```python
from build123d import *

# Parameters (mm, degrees)
F0_W     = 5.2
F0_H     = 1.8
F0_H_2   = 5.2
F0_R     = 1.35
F1_DEPTH = 3
F2_W     = 5.2
F2_H     = 1.8
F3_DEPTH = 1.8
F4_W     = 7
F4_H     = 7
F4_R     = 1.35
F5_DEPTH = 3
F6_R     = 2.5


with BuildPart() as f1:
    # F0 (on Top) → F1 (new body)
    with BuildSketch(Plane.XY):
        with Locations((-0.1, 3.6)):
            Rectangle(F0_W, F0_H)
        Polygon((-4.5, -2.5), (-2.7, -2.5), (-2.7, 2.7), (-2.7, 4.5), (-4.5, 4.5), align=None)
        with Locations((-0.1, 0.1)):
            Rectangle(F0_W, F0_H_2)
        Circle(F0_R, mode=Mode.SUBTRACT)
    extrude(amount=-F1_DEPTH)

    # F0 (on Top) + F2 (on face) → F3 (join)
    with BuildSketch(Plane.XY):
        Polygon((-4.5, -2.5), (-2.7, -2.5), (-2.7, 2.7), (-2.7, 4.5), (-4.5, 4.5), align=None)
    with BuildSketch(Plane.XY):
        with Locations((-0.1, 3.6)):
            Rectangle(F2_W, F2_H)
    extrude(amount=F3_DEPTH)

    # F4 (on face) → F5 (join)
    with BuildSketch(Plane.XY.offset(1.8)):
        with Locations((-1, 1)):
            Rectangle(F4_W, F4_H)
        Circle(F4_R, mode=Mode.SUBTRACT)
    extrude(amount=F5_DEPTH)

    # F6
    f6_edges = [f1.edges().sort_by_distance(p)[0] for p in [
        (2.5, -2.5, 3.3),
        (2.5, -2.5, -1.5),
    ]]
    fillet(f6_edges, radius=F6_R)


solid = f1.part
```
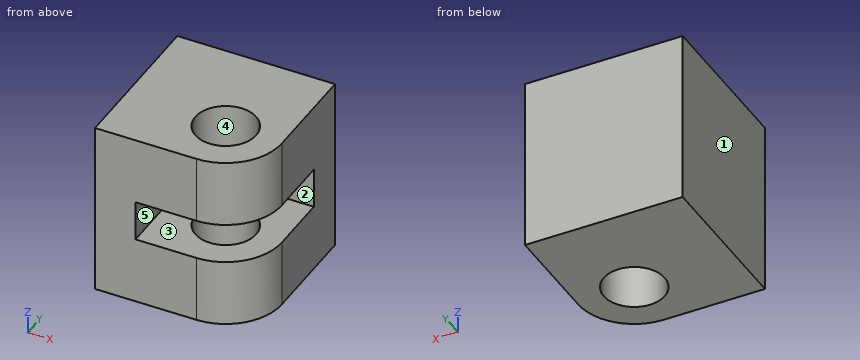
Model file for the job. Use its own axes, mm. Face numbers are marked on the shaded views. A direction names the side the tool comes from. Round coordinates to 2 decimals unless told otherwise and drop trailing zeros. Write each loop counter-clockwise with the first axis right and the second up, starting at its lowest first coordinate (ties: lowest second). Pieces come first, ordered by that corner, then holes. Notation, with made-up numbers: (-6.5, 42) - (34.5, 42) arc R24 ccw to (34.5, 73) - close; hole circle Ø8 at (54, 53.25). An arc over 180 degrees is marked (long way). Use CSV: the item, a comma, the result in double quotes. Start each with the question number.
Item 1: Drill centre lines: L1, parallel to Z at x = 2.25, y = -1; L2, parallel to Y at x = 1.25, z = 1.75; L3, parallel to Y at x = 1, z = 3. Where is each one in solid material? Low to high. Write a range as [from, to].
Item 2: Band-saw the part on C-C (y = 0.75). Write the cut outline in (x, z), and give its area (3 significant figures).
Item 3: Tool access for the marked faces 1 and 2: list every direction of +Z, -Z, +X, -X, +Y, -Y with a clear straight run to the whole face (end or side of a thin tool).
Item 4: Two-plate mould, pull along X, no slides. Class the marked faces 3, 4 and 5: released by +X, released by -X, zero draft, split by the parting line, or undercut.
Item 5: Band-saw the part on D-D (x = 1.5). Write the cut outline in (y, z), and give its area (3 significant figures).
Item 6: Band-saw the part on B-B (x = -0.75). Write the cut outline in (y, z).
Item 7: Band-saw the part on A-A (z = -0.25). Write the cut outline in (x, y), and give its area (3 significant figures).
Item 8: Pin check, flat tips, straight feed: P1, Ø0.9, axis at x = 0, z = 1, coming from the -Y side; P2, Ø0.5, axis at y = 1, z = 1, coming from the +X side. Stop position of each tip, or through.
Checked values:
1,L1,"z = [-3, 0], [1.8, 4.8]"
1,L2,"y = [2.7, 4.5]"
1,L3,"y = [-2.29, -0.91], [0.91, 4.5]"
2,outline,"(-4.5, -3) - (-1.12, -3) - (-1.12, 0) - (-2.7, 0) - (-2.7, 1.8) - (-1.12, 1.8) - (-1.12, 4.8) - (-4.5, 4.8) - close; (1.12, -3) - (2.5, -3) - (2.5, 0) - (1.12, 0) - close; (1.12, 1.8) - (2.5, 1.8) - (2.5, 4.8) - (1.12, 4.8) - close"
2,area,"31.8 mm²"
3,face 1,"+Z, -Z, -X, +Y, -Y"
3,face 2,"+X, -Y"
4,face 3,"zero draft"
4,face 4,"undercut"
4,face 5,"released by +X"
5,outline,"(-2, -3) - (4.5, -3) - (4.5, 4.8) - (-2, 4.8) - (-2, 1.8) - (2.7, 1.8) - (2.7, 0) - (-2, 0) - close"
5,area,"42.2 mm²"
6,outline,"(-2.5, -3) - (-1.12, -3) - (-1.12, 0) - (-2.5, 0) - close; (-2.5, 1.8) - (-1.12, 1.8) - (-1.12, 4.8) - (-2.5, 4.8) - close; (1.12, -3) - (4.5, -3) - (4.5, 4.8) - (1.12, 4.8) - (1.12, 1.8) - (2.7, 1.8) - (2.7, 0) - (1.12, 0) - close"
7,outline,"(-4.5, -2.5) - (0, -2.5) arc R2.5 ccw to (2.5, 0) - (2.5, 4.5) - (-4.5, 4.5) - close; hole circle Ø2.7 at (0, 0)"
7,area,"41.9 mm²"
8,P1,"stops at y = 2.7"
8,P2,"stops at x = -2.7"
